Geometry check sheet. Reference: the model listing, model coordinates, mm. A direction names the side the tool comes from. Round coordinates to 2 decimals unless told otherwise and drop trailing zeros. Loops run counter-clockwise (first coordinate to the right, second up) from the corner with the lowest first, then second, coordinate; pieces in that order, holes last. Notation, with made-up numbers: M 28.5,4 L 52.5,4 A18 ccw 52.5,29 Z; hole C 30.25,71 d3. An arc over 180 degrees is marked long. Use one line per item in the form item = value. Start each with the question number.
1. Material ranges on line 1 (Y direction, x = -40, z = 15.75); line 2 (Z direction, x = -37.5, y = -14.5); line 3 (Y direction, x = 250, z = 9.5), recorded low to high.
2. Cross-section at A-A (x = 0). Record the boundary of the cut face in (y, z), then the cut area to 3 significant figures.
3. Go/stop test with flat-tipped pins: pin 1 (12 mm diameter, centred on x = 86, z = 26.5, fed in from +Y); pin 2 (16 mm diameter, centred on x = -40, y = -26, fed in from -Z); pin 3 (20.5 mm diameter, centred on x = 131, z = 14, fed in from -Y); pin 4 (9 mm diameter, centred on x = 15, y = 43, fed in from -Z). Record where each tip stops, or that it passes through.
4. Cross-section at C-C (x = 157). Record the boundary of the cut face in (y, z), then the cut area to 3 significant figures.
5. Cross-section at B-B (y = -43). Record the boundary of the cut face in (x, z), then the cut area to 3 significant figures.
6. Cross-section at D-D (x = 117). Record the boundary of the cut face in (y, z), then the cut area to 3 significant figures.
7. Set-up check for faces 4 (the cylindrical face through (64, 0, 12)), 5 (the cylindrical face through (104.556, -9.138, -14.416)), 6 (the cylindrical face through (230.749, 10.118, 0.138)), 7 (the cylindrical face through (226, 0, -6)), 8 (the cylindrical face through (-31.485, -0.969, 0.196)): record each of +Z, -Z, +X, -X, +Y, -Y from which the full face is reachable in a straight line by a thin tool's end or side.
8. Draft check along X on faces 1 (the flat face through (32, 1, 21)), 2 (the cylindrical face through (51.013, 11.282, 0.196)), 3 (the cylindrical face through (-48.927, 0.313, -17.451)). Enter one of: pulls with the +X half, pulls with the -X half, needs draft (parallel to the pull), parting line crosses it, or undercut.
```python
from build123d import *

# Parameters (mm, degrees)
SKETCH1_R               = 31.5
SKETCH1_R_2             = 26
BOSS_EXTRUDE1_DEPTH     = 35
SKETCH1_3_R             = 5
SKETCH1_3_R_2           = 31.5
BOSS_EXTRUDE2_DEPTH     = 21
BOSS_EXTRUDE3_DEPTH     = 2.5
CUT_EXTRUDE1_DEPTH      = 250.214133183
CUT_EXTRUDE1_DEPTH_BACK = 250.214133183
SKETCH1_5_R             = 17.5
SKETCH1_5_R_2           = 12
BOSS_EXTRUDE4_DEPTH     = 21
CUT_EXTRUDE2_DEPTH      = 14


with BuildPart() as part:
    # Sketch1 → Boss-Extrude1 (new, symmetric)
    with BuildSketch(Plane.XY):
        Circle(SKETCH1_R)
        Circle(SKETCH1_R_2, mode=Mode.SUBTRACT)
    extrude(amount=BOSS_EXTRUDE1_DEPTH, both=True)

    # Sketch1_3 → Boss-Extrude2 (add, symmetric)
    with BuildSketch(Plane.XY):
        with BuildLine():
            Line((220, 8.719912605), (87.482015231, 12.190018161))
            ThreePointArc((87.482015231, 12.190018161), (51.997088566, 22.622612499), (26.373739078, 49.29587638))
            ThreePointArc((26.373739078, 49.29587638), (17.709961948, 55.714405462), (7.181946677, 53.386435492))
            ThreePointArc((7.181946677, 53.386435492), (-14.855989459, 42.122318837), (-39.406288617, 38.986435492))
            ThreePointArc((-39.406288617, 38.986435492), (-50.326951915, 33.896458963), (-52.376901133, 22.023529412))
            ThreePointArc((-52.376901133, 22.023529412), (-48.925892025, 0), (-52.376901133, -22.023529412))
            ThreePointArc((-52.376901133, -22.023529412), (-50.326951915, -33.896458963), (-39.406288617, -38.986435492))
            ThreePointArc((-39.406288617, -38.986435492), (-14.855989459, -42.122318837), (7.181946677, -53.386435492))
            ThreePointArc((7.181946677, -53.386435492), (17.709961948, -55.714405462), (26.373739078, -49.29587638))
            ThreePointArc((26.373739078, -49.29587638), (51.997088566, -22.622612499), (87.482015231, -12.190018161))
            Line((87.482015231, -12.190018161), (220, -8.719912605))
            ThreePointArc((220, -8.719912605), (230.604685788, -10.075596562), (240.30539773, -14.569306326))
            ThreePointArc((240.30539773, -14.569306326), (232.5, 0), (240.30539773, 14.569306326))
            ThreePointArc((240.30539773, 14.569306326), (230.604685788, 10.075596562), (220, 8.719912605))
        make_face()
        with Locations(Location((15, -43, 0), (0, 0, 180))):
            Circle(SKETCH1_3_R, mode=Mode.SUBTRACT)
        with Locations(Location((-40, -26, 0), (0, 0, 180))):
            Circle(SKETCH1_3_R, mode=Mode.SUBTRACT)
        Circle(SKETCH1_3_R_2, mode=Mode.SUBTRACT)
        with Locations(Location((-40, 26, 0), (0, 0, 180))):
            Circle(SKETCH1_3_R, mode=Mode.SUBTRACT)
        with Locations(Location((15, 43, 0), (0, 0, 180))):
            Circle(SKETCH1_3_R, mode=Mode.SUBTRACT)
        with BuildLine():
            ThreePointArc((70, -6), (64, 0), (70, 6))
            Line((70, 6), (220, 6))
            ThreePointArc((220, 6), (226, 0), (220, -6))
            Line((220, -6), (70, -6))
        make_face(mode=Mode.SUBTRACT)
    extrude(amount=BOSS_EXTRUDE2_DEPTH, both=True)

    # Sketch1_4 → Boss-Extrude3 (add, symmetric)
    with BuildSketch(Plane.XY):
        with BuildLine():
            Line((70, -6), (220, -6))
            ThreePointArc((220, -6), (226, 0), (220, 6))
            Line((220, 6), (70, 6))
            ThreePointArc((70, 6), (64, 0), (70, -6))
        make_face()
    extrude(amount=BOSS_EXTRUDE3_DEPTH, both=True)

    # Sketch2 → Cut-Extrude1 (cut, two sides: drawn at the far end of the back side and taken through both)
    with BuildSketch(Plane(origin=(0, 0, 0), x_dir=(1, 0, 0), z_dir=(0, 1, 0)).offset(-CUT_EXTRUDE1_DEPTH_BACK)):
        with BuildLine():
            Line((240.30539773, -9.422684737), (122.188711449, -12))
            ThreePointArc((122.188711449, -12), (104.311213199, -14.478720031), (87.482015231, -21))
            Line((87.482015231, -21), (240.30539773, -21))
            Line((240.30539773, -21), (240.30539773, -9.422684737))
        make_face()
        with BuildLine():
            Line((240.30539773, 9.422684737), (122.188711449, 12))
            ThreePointArc((122.188711449, 12), (104.311213199, 14.478720031), (87.482015231, 21))
            Line((87.482015231, 21), (240.30539773, 21))
            Line((240.30539773, 21), (240.30539773, 9.422684737))
        make_face()
    extrude(amount=CUT_EXTRUDE1_DEPTH + CUT_EXTRUDE1_DEPTH_BACK, mode=Mode.SUBTRACT)

    # Sketch1_5 → Boss-Extrude4 (add, symmetric)
    with BuildSketch(Plane.XY):
        with Locations((250, 0)):
            Circle(SKETCH1_5_R)
        with Locations(Location((250, 0, 0), (0, 0, 180))):
            Circle(SKETCH1_5_R_2, mode=Mode.SUBTRACT)
    extrude(amount=BOSS_EXTRUDE4_DEPTH, both=True)

    # Sketch3 → Cut-Extrude2 (cut, symmetric)
    with BuildSketch(Plane.XY):
        with BuildLine():
            ThreePointArc((18.496414213, 25.497699136), (51.511708097, 11.184621648), (87.482015231, 12.190018161))
            ThreePointArc((87.482015231, 12.190018161), (51.997088566, 22.622612499), (26.373739078, 49.29587638))
            ThreePointArc((26.373739078, 49.29587638), (17.709961948, 55.714405462), (7.181946677, 53.386435492))
            ThreePointArc((7.181946677, 53.386435492), (-14.855989459, 42.122318837), (-39.406288617, 38.986435492))
            ThreePointArc((-39.406288617, 38.986435492), (-50.326951915, 33.896458963), (-52.376901133, 22.023529412))
            ThreePointArc((-52.376901133, 22.023529412), (-48.925892025, 0), (-52.376901133, -22.023529412))
            ThreePointArc((-52.376901133, -22.023529412), (-50.326951915, -33.896458963), (-39.406288617, -38.986435492))
            ThreePointArc((-39.406288617, -38.986435492), (-14.855989459, -42.122318837), (7.181946677, -53.386435492))
            ThreePointArc((7.181946677, -53.386435492), (17.709961948, -55.714405462), (26.373739078, -49.29587638))
            ThreePointArc((26.373739078, -49.29587638), (51.997088566, -22.622612499), (87.482015231, -12.190018161))
            ThreePointArc((87.482015231, -12.190018161), (51.511708097, -11.184621648), (18.496414213, -25.497699136))
            ThreePointArc((18.496414213, -25.497699136), (-31.5, 0), (18.496414213, 25.497699136))
        make_face()
    extrude(amount=CUT_EXTRUDE2_DEPTH, both=True, mode=Mode.SUBTRACT)


solid = part.part
```
Reported:
q1.line_1 = -39 to -31, -21 to 21, 31 to 39
q1.line_2 = -21 to -14, 14 to 21
q1.line_3 = -17.5 to -12, 12 to 17.5
q2.outline = M -48.63,-21 L -31.5,-21 L -31.5,-35 L -26,-35 L -26,35 L -31.5,35 L -31.5,21 L -48.63,21 L -48.63,14 L -31.5,14 L -31.5,-14 L -48.63,-14 Z; M 26,-35 L 31.5,-35 L 31.5,-21 L 48.63,-21 L 48.63,-14 L 31.5,-14 L 31.5,14 L 48.63,14 L 48.63,21 L 31.5,21 L 31.5,35 L 26,35 Z
q2.area = 1,250 mm²
q3.pin_1 = 12.4
q3.pin_2 = -21
q3.pin_3 = -11.31
q3.pin_4 = through
q4.outline = M -10.37,-11.24 L -6,-11.24 L -6,-2.5 L 6,-2.5 L 6,-11.24 L 10.37,-11.24 L 10.37,11.24 L 6,11.24 L 6,2.5 L -6,2.5 L -6,11.24 L -10.37,11.24 Z
q4.area = 256 mm²
q5.outline = M -12.2,-21 L 10,-21 L 10,-14 L -12.2,-14 Z; M -12.2,14 L 10,14 L 10,21 L -12.2,21 Z; M 20,-21 L 30.3,-21 L 30.3,-14 L 20,-14 Z; M 20,14 L 30.3,14 L 30.3,21 L 20,21 Z
q5.area = 455 mm²
q6.outline = M -11.42,-12.29 L -6,-12.29 L -6,-2.5 L 6,-2.5 L 6,-12.29 L 11.42,-12.29 L 11.42,12.29 L 6,12.29 L 6,2.5 L -6,2.5 L -6,12.29 L -11.42,12.29 Z
q6.area = 326 mm²
q7.face_4 = +Z
q7.face_5 = -Z, +Y, -Y
q7.face_6 = +Z, -Z, +Y
q7.face_7 = -Z
q7.face_8 = none
q8.face_1 = needs draft
q8.face_2 = undercut
q8.face_3 = pulls with the -X half
